from build123d import *

# Parameters (mm, degrees)
SKETCH1_R               = 10
SKETCH1_R_2             = 5
BOSS_EXTRUDE1_DEPTH     = 1.5
SKETCH3_R               = 1
ALIGNMENTHOLE_CUT_DEPTH = 15.456832295
CIRPATTERN1_COUNT       = 2


with BuildPart() as part:
    # Sketch1 → Boss-Extrude1 (new, symmetric)
    with BuildSketch(Plane.XY):
        Circle(SKETCH1_R)
        Circle(SKETCH1_R_2, mode=Mode.SUBTRACT)
    extrude(amount=BOSS_EXTRUDE1_DEPTH, both=True)

    # Sketch3 → AlignmentHole-Cut (cut, through all)
    with BuildSketch(Plane.XY.offset(1.5)):
        with Locations((-7, 0)):
            Circle(SKETCH3_R)
    alignmenthole_cut = extrude(amount=-ALIGNMENTHOLE_CUT_DEPTH, mode=Mode.SUBTRACT)

    # CirPattern1: AlignmentHole-Cut ×2 about axis
    cirpattern1_axis = Axis((0, 0, 0), (0, 0, 1))
    for i in range(1, CIRPATTERN1_COUNT):
        add(alignmenthole_cut.rotate(cirpattern1_axis, i * 360 / CIRPATTERN1_COUNT), mode=Mode.SUBTRACT)


solid = part.part
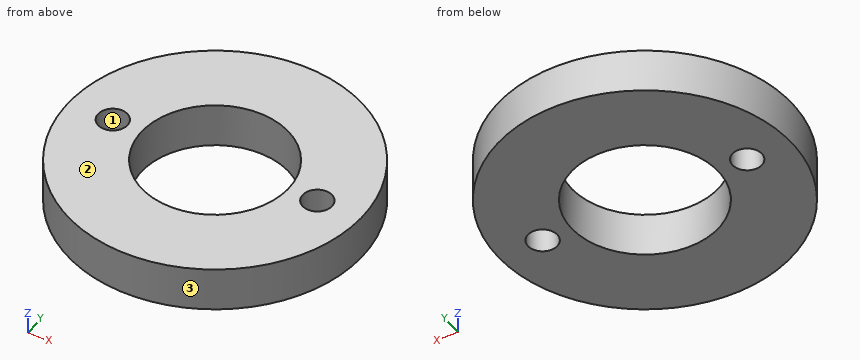
Could you check a few things on this model? Use its own coordinates, in mm. Face numbers are marked on the shaded views. Coordinates: 2 decimals unless noted, no trailing zeros. Order: outer loops, then holes, each group sorted by start corner. A loop starts at its lowest first (then second) coordinate and runs counter-clockwise, first axis right, second up.
Q1. Suppose I cut it at B-B on x = 0. Please give me the cut outline in (y, z), and give its area (3 significant figures).
Q2. Suppose I cut it at D-D on x = -7.75. Please give me the cut outline in (y, z), and give its area (3 significant figures).
Q3. Suppose I cut it at C-C on z = -1. Please give me the cut outline in (x, y), and give its area (3 significant figures).
Q4. Will these pins go through, and if not, where does the flat tip stop? pin 1 (3 mm diameter, centred on x = 7, y = 0, fed in from +Z); pin 2 (1.5 mm diameter, centred on x = -6.5, z = 0, fed in from -Y).
Q5. Suppose I cut it at A-A on y = 0. Please give me the cut outline in (x, z).
Q6. Thinking about a two-plate mould opening in X: for the marked faces 1, 2 and 3, which applies, released by +X, released by -X, zero draft, split by the parting line, or undercut?
Q7. Please list where these lines run through material, in increasing order: L1, parallel to X at y = -0.5, z = 0.25; L2, parallel to Y at x = 0, z = 0.1; L3, parallel to Y at x = 3.5, z = 0.5.
Answer:
1. outline: (-10, -1.5) - (-5, -1.5) - (-5, 1.5) - (-10, 1.5) - close; (5, -1.5) - (10, -1.5) - (10, 1.5) - (5, 1.5) - close
1. area: 30.0 mm2
2. outline: (-6.32, -1.5) - (-0.66, -1.5) - (-0.66, 1.5) - (-6.32, 1.5) - close; (0.66, -1.5) - (6.32, -1.5) - (6.32, 1.5) - (0.66, 1.5) - close
2. area: 33.9 mm2
3. outline: circle Ø20 at (0, 0); hole circle Ø2 at (-7, 0); hole circle Ø10 at (0, 0); hole circle Ø2 at (7, 0)
3. area: 229 mm2
4. pin 1: stops at z = 1.5
4. pin 2: stops at y = -8.18
5. outline: (-10, -1.5) - (-8, -1.5) - (-8, 1.5) - (-10, 1.5) - close; (-6, -1.5) - (-5, -1.5) - (-5, 1.5) - (-6, 1.5) - close; (5, -1.5) - (6, -1.5) - (6, 1.5) - (5, 1.5) - close; (8, -1.5) - (10, -1.5) - (10, 1.5) - (8, 1.5) - close
6. face 1: undercut
6. face 2: zero draft
6. face 3: split by the parting line
7. L1: x = -9.99 to -7.87, -6.13 to -4.97, 4.97 to 6.13, 7.87 to 9.99
7. L2: y = -10 to -5, 5 to 10
7. L3: y = -9.37 to -3.57, 3.57 to 9.37
